Could you check a few things on this model? Use its own coordinates, in mm. Face numbers are marked on the shaded views. A direction names the side the tool comes from. Coordinates: 2 decimals unless noted, no trailing zeros. Write each loop counter-clockwise with the first axis right and the second up, starting at its lowest first coordinate (ties: lowest second). Pieces come first, ordered by that corner, then holes. Notation, with made-up numbers: (63.25, 18) - (109.25, 18) arc R19 cw to (109.25, 46) - close; hole circle Ø3 at (3, 10.25). An arc over 180 degrees is marked (long way). Write item = value, one per line. Start each with the question number.
```python
from build123d import *

# Parameters (mm, degrees)
F1_DEPTH = 3.4925
F3_R     = 9.525
F4_DEPTH = 4.191


with BuildPart() as f1:
    # F0 (on Top) → F1 (new body, symmetric)
    with BuildSketch(Plane.XY):
        with BuildLine():
            ThreePointArc((0, 11.00455), (-7.781392, -7.781392), (11.00455, 0))
            ThreePointArc((11.00455, 0), (7.781392, 7.781392), (0, 11.00455))
        make_face()
        with BuildLine():
            Line((12.7, 12.7), (0, 12.7))
            Line((0, 12.7), (-12.7, 12.7))
            ThreePointArc((-12.7, 12.7), (-13.945568, 8.051477), (-17.348523, 4.648523))
            Line((-17.348523, 4.648523), (-4.648523, -17.348523))
            ThreePointArc((-4.648523, -17.348523), (0, -16.102955), (4.648523, -17.348523))
            Line((4.648523, -17.348523), (17.348523, 4.648523))
            ThreePointArc((17.348523, 4.648523), (13.945568, 8.051477), (12.7, 12.7))
        make_face()
        with BuildLine():
            ThreePointArc((0, 11.00455), (7.781392, 7.781392), (11.00455, 0))
            ThreePointArc((11.00455, 0), (-7.781392, -7.781392), (0, 11.00455))
        make_face(mode=Mode.SUBTRACT)
        with BuildLine():
            Line((-12.7, 12.7), (0, 12.7))
            Line((0, 12.7), (12.7, 12.7))
            Line((12.7, 12.7), (12.7, 34.925))
            ThreePointArc((12.7, 34.925), (11.770064, 37.170064), (9.525, 38.1))
            Line((9.525, 38.1), (-9.525, 38.1))
            ThreePointArc((-9.525, 38.1), (-11.770064, 37.170064), (-12.7, 34.925))
            Line((-12.7, 34.925), (-12.7, 12.7))
        make_face()
        with BuildLine():
            Line((-4.648523, -17.348523), (-17.348523, 4.648523))
            Line((-17.348523, 4.648523), (-36.595937, -6.463977))
            ThreePointArc((-36.595937, -6.463977), (-38.075252, -8.391858), (-37.758068, -10.801108))
            Line((-37.758068, -10.801108), (-28.233068, -27.298892))
            ThreePointArc((-28.233068, -27.298892), (-26.305188, -28.778206), (-23.895937, -28.461023))
            Line((-23.895937, -28.461023), (-4.648523, -17.348523))
        make_face()
        with BuildLine():
            Line((36.595937, -6.463977), (17.348523, 4.648523))
            Line((17.348523, 4.648523), (4.648523, -17.348523))
            Line((4.648523, -17.348523), (23.895937, -28.461023))
            ThreePointArc((23.895937, -28.461023), (26.305188, -28.778206), (28.233068, -27.298892))
            Line((28.233068, -27.298892), (37.758068, -10.801108))
            ThreePointArc((37.758068, -10.801108), (38.075252, -8.391858), (36.595937, -6.463977))
        make_face()
    extrude(amount=F1_DEPTH, both=True)

    # F3 (on face) → F4 (cut)
    with BuildSketch(Plane(origin=(0, 0, -3.4925), x_dir=(1, 0, 0), z_dir=(0, 0, -1))):
        with Locations((0, -25.4)):
            Circle(F3_R)
        with Locations((21.997045, 12.7)):
            Circle(F3_R)
        with Locations((-21.997045, 12.7)):
            Circle(F3_R)
    extrude(amount=-F4_DEPTH, mode=Mode.SUBTRACT)


solid = f1.part
```
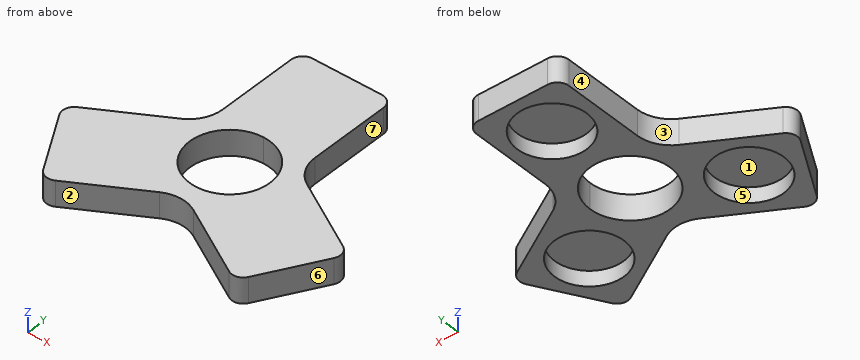
1) Suppose I cut it at C-C on z = 2.5. Please give me the cut outline in (x, y) (3 decimals).
2) Which directions (+Z, -Z, +X, -X, +Y, -Y) give clear straight access to the entire face, cutting with the end or side of a thin tool? Please do the marked faces 4, 5, 6 and 7.
3) For P1, Ø2, axis at y = -10.5, z = -0.5, coming from the -X side; P2, Ø1, axis at y = 15, z = 1.5, coming from the +X side; P3, Ø8, axis at x = 1, y = -6, coming from the -Z side; P4, Ø5.5, axis at x = -19.5, y = -16, coming from the -Z side, each with a flat end and sliding along its axis, tell me the tip position at first contact or that it passes through.
4) Suppose I cut it at D-D on x = -25. Please give me the cut outline in (y, z).
5) If I drill on probe 1 along Y at (x, z) = (0, -0.9) (3 decimals); probe 2 along X at (y, z) = (25.4, -1.1) (3 decimals); probe 3 along X at (y, z) = (-4, -1), over which ranges is the centre line in solid material (lowest first)? Write a range as [from, to].
6) Suppose I cut it at B-B on z = -1.25. Please give me the cut outline in (x, y) (3 decimals), plus the area to 3 significant figures.
7) Thinking about a two-plate mould opening in Y: for the marked faces 1, 2 and 3, which applies, +Y half, -Y half, draft (parallel to the pull), parting line (faces both ways), or undercut?
8) Suppose I cut it at A-A on y = 2. Please give me the cut outline in (x, z).
Reply:
q1.outline = (-37.758, -10.801) - (-28.233, -27.299) arc R3.175 ccw to (-23.896, -28.461) - (-4.649, -17.349) arc R9.297 cw to (4.649, -17.349) - (23.896, -28.461) arc R3.175 ccw to (28.233, -27.299) - (37.758, -10.801) arc R3.175 ccw to (36.596, -6.464) - (17.349, 4.649) arc R9.297 cw to (12.7, 12.7) - (12.7, 34.925) arc R3.175 ccw to (9.525, 38.1) - (-9.525, 38.1) arc R3.175 ccw to (-12.7, 34.925) - (-12.7, 12.7) arc R9.297 cw to (-17.349, 4.649) - (-36.596, -6.464) arc R3.175 ccw to start; hole circle Ø22.009 at (0, 0)
q2.face_4 = +Z, -Z, -X, +Y
q2.face_5 = -Z
q2.face_6 = +Z, -Z, +X, -Y
q2.face_7 = +Z, -Z, +X, +Y
q3.P1 = -38.17
q3.P2 = 12.7
q3.P3 = through
q3.P4 = 0.7
q4.outline = (-28.85, -3.49) - (-21.74, -3.49) - (-21.74, 0.7) - (-3.66, 0.7) - (-3.66, -3.49) - (0.23, -3.49) - (0.23, 3.49) - (-28.85, 3.49) - close
q5.probe_1 = [-16.103, -11.005], [11.005, 15.875], [34.925, 38.1]
q5.probe_2 = [-12.7, -9.525], [9.525, 12.7]
q5.probe_3 = [-32.33, -25.87], [-18.12, -10.25], [10.25, 18.12], [25.87, 32.33]
q6.outline = (-37.758, -10.801) - (-28.233, -27.299) arc R3.175 ccw to (-23.896, -28.461) - (-4.649, -17.349) arc R9.297 cw to (4.649, -17.349) - (23.896, -28.461) arc R3.175 ccw to (28.233, -27.299) - (37.758, -10.801) arc R3.175 ccw to (36.596, -6.464) - (17.349, 4.649) arc R9.297 cw to (12.7, 12.7) - (12.7, 34.925) arc R3.175 ccw to (9.525, 38.1) - (-9.525, 38.1) arc R3.175 ccw to (-12.7, 34.925) - (-12.7, 12.7) arc R9.297 cw to (-17.349, 4.649) - (-36.596, -6.464) arc R3.175 ccw to start; hole circle Ø19.05 at (-21.997, -12.7); hole circle Ø22.009 at (0, 0); hole circle Ø19.05 at (0, 25.4); hole circle Ø19.05 at (21.997, -12.7)
q6.area = 1,390 mm^2
q7.face_1 = undercut
q7.face_2 = -Y half
q7.face_3 = +Y half
q8.outline = (-21.94, -3.49) - (-10.82, -3.49) - (-10.82, 3.49) - (-21.94, 3.49) - close; (10.82, -3.49) - (21.94, -3.49) - (21.94, 3.49) - (10.82, 3.49) - close
